Verification items for the finished model (mm, model axes). A direction names the side the tool comes from. Give positions to 0.01 mm unless a question says otherwise; leave off trailing zeros. Write each loop counter-clockwise with the first axis right and the second up, starting at its lowest first coordinate (ties: lowest second). Pieces come first, ordered by that corner, then holes.
from build123d import *

# Parameters (mm, degrees)
F0_W     = 420
F0_H     = 297
F1_DEPTH = 18
F2_DEPTH = 25


with BuildPart() as f1:
    # F0 (on Top) → F1 (new body)
    with BuildSketch(Plane.XY):
        with BuildLine():
            Line((36.669135, 748.890698), (-613.330865, 748.890698))
            Line((-613.330865, 748.890698), (-613.330865, -31.109302))
            ThreePointArc((-613.330865, -31.109302), (-578.183679, -115.962116), (-493.330865, -151.109302))
            Line((-493.330865, -151.109302), (-83.330865, -151.109302))
            ThreePointArc((-83.330865, -151.109302), (1.521949, -115.962116), (36.669135, -31.109302))
            Line((36.669135, -31.109302), (36.669135, 748.890698))
        make_face()
        with Locations((-288.491384, 32.537884)):
            Rectangle(F0_W, F0_H, mode=Mode.SUBTRACT)
    extrude(amount=F1_DEPTH)

    # F0 (on Top) → F2 (join)
    with BuildSketch(Plane.XY):
        with BuildLine():
            Line((36.669135, 748.890698), (-613.330865, 748.890698))
            Line((-613.330865, 748.890698), (-613.330865, -31.109302))
            ThreePointArc((-613.330865, -31.109302), (-578.183679, -115.962116), (-493.330865, -151.109302))
            Line((-493.330865, -151.109302), (-83.330865, -151.109302))
            ThreePointArc((-83.330865, -151.109302), (1.521949, -115.962116), (36.669135, -31.109302))
            Line((36.669135, -31.109302), (36.669135, 748.890698))
        make_face()
        with Locations((-288.491384, 32.537884)):
            Rectangle(F0_W, F0_H, mode=Mode.SUBTRACT)
    extrude(amount=F2_DEPTH)


solid = f1.part
Item 1: Scan lines: line 1 along Y through (x, z) = (-250, 20.5); line 2 along X through (y, z) = (-4.5, 16.5); line 3 along X through (y, z) = (-77, 4.5). Record each from-to range of solid material in increasing order.
Answer key:
line 1: y = -151.11 to -115.96, 181.04 to 748.89
line 2: x = -613.33 to -498.49, -78.49 to 36.67
line 3: x = -604.21 to -498.49, -78.49 to 27.55
Item 2: Sectioned sample at C-C on y = -44. Record the cut outline in (x, z), then the cut area to 3 significant figures.
Answer key:
outline: (-612.64, 0) - (-498.49, 0) - (-498.49, 25) - (-612.64, 25) - close; (-78.49, 0) - (35.97, 0) - (35.97, 25) - (-78.49, 25) - close
area: 5,720 mm2
Item 3: Set-up check for faces 1 (the face through (-291, 181.038, 12)), 2 (the face through (0.584, -116.89, 12.325)): record each of +Z, -Z, +X, -X, +Y, -Y from which the full face is reachable in a straight line by a thin tool's end or side.
Answer key:
face 1: +Z, -Z
face 2: +Z, -Z, +X, -Y
Item 4: Depth check by flat-ended pin: pin 1 (1.5 mm diameter, centred on x = -515.5, y = 184, fed in from -Z). Enter the tip coordinate at first touch or a pass-through.
Answer key:
pin 1: stops at z = 0
Item 5: Sectioned sample at A-A on x = -319. Record the cut outline in (y, z).
Answer key:
outline: (-151.11, 0) - (-115.96, 0) - (-115.96, 25) - (-151.11, 25) - close; (181.04, 0) - (748.89, 0) - (748.89, 25) - (181.04, 25) - close
Item 6: Release check for a two-part mould opening along Y. For faces 3 (the face through (-291, -115.962, 12)), 4 (the face through (-579.112, -115.024, 12.325)), 5 (the face through (-78.491, 30, 12)), 6 (the face through (-293, 405, 0)) record: released by +Y, released by -Y, zero draft, split by the parting line, or undercut.
Answer key:
face 3: undercut
face 4: released by -Y
face 5: undercut
face 6: zero draft
Item 7: Sectioned sample at B-B on z = 4.5. Record the cut outline in (x, y), then the cut area to 3 significant figures.
Answer key:
outline: (-613.33, -31.11) arc R120 ccw to (-493.33, -151.11) - (-83.33, -151.11) arc R120 ccw to (36.67, -31.11) - (36.67, 748.89) - (-613.33, 748.89) - close; hole (-498.49, -115.96) - (-78.49, -115.96) - (-78.49, 181.04) - (-498.49, 181.04) - close
area: 454,000 mm2
